CAD build for the part. Positions are in the model's coordinates, mm. A direction names the side the tool comes from. Coordinates: 2 decimals unless noted, no trailing zeros.
from build123d import *

# Parameters (mm, degrees)
SKIZZE2_W                            = 24
SKIZZE2_H                            = 26
SCHNITT_LINEAR_AUSTRAGEN1_DEPTH      = 62.5
KREISMUSTER1_COUNT                   = 8
SKIZZE3_R                            = 1.65
SCHNITT_LINEAR_AUSTRAGEN2_DEPTH      = 29.067398613
KREISMUSTER2_COUNT                   = 8
SKIZZE4_R                            = 1.25
SCHNITT_LINEAR_AUSTRAGEN3_DEPTH      = 6
SCHNITT_LINEAR_AUSTRAGEN3_DEPTH_BACK = 27.0000001
SCHNITT_LINEAR_AUSTRAGEN4_REACH      = 42
SKIZZE5_W                            = 3
SKIZZE5_H                            = 36.82390528
SKIZZE6_W                            = 7.166939891
SKIZZE6_H                            = 30
SCHNITT_LINEAR_AUSTRAGEN5_DEPTH      = 2.0000001
SCHNITT_LINEAR_AUSTRAGEN5_DEPTH_BACK = 2.5
SKIZZE12_R                           = 1.25
SCHNITT_LINEAR_AUSTRAGEN6_DEPTH      = 10
SCHNITT_LINEAR_AUSTRAGEN7_REACH      = 39.5


with BuildPart() as part:
    # Skizze1 → Rotation1 (revolve)
    with BuildSketch(Plane.XY):
        Polygon((-53, -1), (-53, 40), (-60, 40), (-60, 11), (-61.5, 11), (-61.5, 8), (-55, 8), (-55, 3.600622615), (-58, 1.5), (-58, 0), (-54, 0), (-54, -1), align=None)
    revolve(axis=Axis((0, 0, 0), (0, 1, 0)))

    # Skizze2 → Schnitt-Linear austragen1 (cut, through all)
    with BuildSketch(Plane(origin=(0, 0, 0), x_dir=(0, 0, -1), z_dir=(1, 0, 0))):
        with Locations((0, 27)):
            Rectangle(SKIZZE2_W, SKIZZE2_H)
    schnitt_linear_austragen1 = extrude(amount=-SCHNITT_LINEAR_AUSTRAGEN1_DEPTH, mode=Mode.SUBTRACT)

    # Kreismuster1: Schnitt-Linear austragen1 ×8 about axis
    kreismuster1_axis = Axis((0, 0, 0), (0, 1, 0))
    for i in range(1, KREISMUSTER1_COUNT):
        add(schnitt_linear_austragen1.rotate(kreismuster1_axis, i * 360 / KREISMUSTER1_COUNT), mode=Mode.SUBTRACT)

    # Skizze3 → Schnitt-Linear austragen2 (cut, through all)
    with BuildSketch(Plane(origin=(20.009071561, 0, 48.306171934), x_dir=(-0.923879533, 0, 0.382683432), z_dir=(-0.382683432, 0, -0.923879533))):
        with Locations((0, 25)):
            Circle(SKIZZE3_R)
    schnitt_linear_austragen2 = extrude(amount=-SCHNITT_LINEAR_AUSTRAGEN2_DEPTH, mode=Mode.SUBTRACT)

    # Kreismuster2: Schnitt-Linear austragen2 ×8 about axis
    kreismuster2_axis = Axis((0, 0, 0), (0, -1, 0))
    for i in range(1, KREISMUSTER2_COUNT):
        add(schnitt_linear_austragen2.rotate(kreismuster2_axis, i * 360 / KREISMUSTER2_COUNT), mode=Mode.SUBTRACT)

    # Skizze4 → Schnitt-Linear austragen3 (cut, two sides)
    with BuildSketch(Plane(origin=(0, 14, 0), x_dir=(-1, 0, 0), z_dir=(0, -1, 0))) as schnitt_linear_austragen3_sk:
        with Locations((0, 57)):
            Circle(SKIZZE4_R)
        with Locations((40.305086528, 40.305086528)):
            Circle(SKIZZE4_R)
        with Locations((57, 0)):
            Circle(SKIZZE4_R)
        with Locations((40.305086528, -40.305086528)):
            Circle(SKIZZE4_R)
        with Locations((0, -57)):
            Circle(SKIZZE4_R)
        with Locations((-40.305086528, -40.305086528)):
            Circle(SKIZZE4_R)
        with Locations((-57, 0)):
            Circle(SKIZZE4_R)
        with Locations((-40.305086528, 40.305086528)):
            Circle(SKIZZE4_R)
    extrude(amount=SCHNITT_LINEAR_AUSTRAGEN3_DEPTH, mode=Mode.SUBTRACT)
    extrude(schnitt_linear_austragen3_sk.sketch, amount=-SCHNITT_LINEAR_AUSTRAGEN3_DEPTH_BACK, mode=Mode.SUBTRACT)

    # Skizze5 → Schnitt-Linear austragen4 (cut, up to next)
    with BuildSketch(Plane.XZ, mode=Mode.PRIVATE) as schnitt_linear_austragen4_sk1:
        with Locations((56.5, 0)):
            Rectangle(SKIZZE5_W, SKIZZE5_H)
    schnitt_linear_austragen4_tool1 = extrude(schnitt_linear_austragen4_sk1.sketch, amount=-SCHNITT_LINEAR_AUSTRAGEN4_REACH, mode=Mode.PRIVATE) & part.part
    add(schnitt_linear_austragen4_tool1.solids().sort_by_distance((56.5, 0, 0))[0], mode=Mode.SUBTRACT)

    # Skizze6 → Schnitt-Linear austragen5 (cut, two sides)
    with BuildSketch(Plane.XZ) as schnitt_linear_austragen5_sk:
        with Locations((-54.416530055, 0)):
            Rectangle(SKIZZE6_W, SKIZZE6_H)
    extrude(amount=SCHNITT_LINEAR_AUSTRAGEN5_DEPTH, mode=Mode.SUBTRACT)
    extrude(schnitt_linear_austragen5_sk.sketch, amount=-SCHNITT_LINEAR_AUSTRAGEN5_DEPTH_BACK, mode=Mode.SUBTRACT)

    # Skizze12 → Schnitt-Linear austragen6 (cut)
    with BuildSketch(Plane(origin=(0, 40, 0), x_dir=(1, 0, 0), z_dir=(0, 1, 0))):
        with Locations((-51.737253821, -21.430272212)):
            Circle(SKIZZE12_R)
        with Locations((-51.737253821, 21.430272212)):
            Circle(SKIZZE12_R)
        with Locations((-21.430272212, 51.737253821)):
            Circle(SKIZZE12_R)
        with Locations((21.430272212, 51.737253821)):
            Circle(SKIZZE12_R)
        with Locations((51.737253821, 21.430272212)):
            Circle(SKIZZE12_R)
        with Locations((51.737253821, -21.430272212)):
            Circle(SKIZZE12_R)
        with Locations((21.430272212, -51.737253821)):
            Circle(SKIZZE12_R)
        with Locations((-21.430272212, -51.737253821)):
            Circle(SKIZZE12_R)
    extrude(amount=-SCHNITT_LINEAR_AUSTRAGEN6_DEPTH, mode=Mode.SUBTRACT)

    # Skizze13 → Schnitt-Linear austragen7 (cut, up to next)
    with BuildSketch(Plane.XZ.offset(-2.5), mode=Mode.PRIVATE) as schnitt_linear_austragen7_sk1:
        with BuildLine():
            Line((-53.5, -5), (-53.5, 5))
            ThreePointArc((-53.5, 5), (-49.5, 9), (-45.5, 5))
            Line((-45.5, 5), (-45.5, -5))
            ThreePointArc((-45.5, -5), (-49.5, -9), (-53.5, -5))
        make_face()
    schnitt_linear_austragen7_tool1 = extrude(schnitt_linear_austragen7_sk1.sketch, amount=-SCHNITT_LINEAR_AUSTRAGEN7_REACH, mode=Mode.PRIVATE) & part.part
    add(schnitt_linear_austragen7_tool1.solids().sort_by_distance((-49.5, 2.5, 0))[0], mode=Mode.SUBTRACT)


solid = part.part
1) Drill centre lines: probe 1 along Z at (x, y) = (20.5, 34); probe 2 along Y at (x, z) = (-40.5, 34.5); probe 3 along Y at (x, z) = (-1.5, -54.5). Where is each one in solid material? Low to high.
2) Pin check, flat tips, straight feed: P1, Ø2, axis at y = 24, z = 47.5, coming from the +X side; P2, Ø12, axis at y = 21, z = 12.5, coming from the -X side; P3, Ø3, axis at x = 22, y = 5.5, coming from the -Z side. Stop position of each tip, or through.
3) Which spindle directions (+Z, -Z, +X, -X, +Y, -Y) get a long thin tool onto all of the face, cutting with end or side? Do faces 1 (the flat face through (-12, 27, -55)), 2 (the flat face through (-54, 2.5, 0)), 3 (the flat face through (55, 1, 0)), 4 (the flat face through (-50, 0, -21)). Say none if no direction does.
4) Two-plate mould, pull along Z, no slides. Class faces 5 (the cylindrical face through (-28.38, 9.48, -54.56)), 6 (the flat face through (20, 40, -52)), 7 (the flat face through (-55, 14, 0)): released by +Z, released by -Z, zero draft, split by the parting line, or undercut.
5) Slice it at A-A (y = 21.5). Give the number of separate pieces and of enclosed holes in the cut face, plus the area to 3 significant figures.
Worked out:
1. probe 1: z = -56.39 to -52.57, -50.9 to -48.87, 48.87 to 50.9, 52.57 to 56.39
1. probe 2: y = -1 to 14
1. probe 3: y = 0 to 14
2. P1: stops at x = 31.53
2. P2: stops at x = -58.79
2. P3: stops at z = -51.04
3. face 1: +Z, -Z, +Y
3. face 2: -X, -Y
3. face 3: +Z, -Z, +X, -Y
3. face 4: -Y
4. face 5: split by the parting line
4. face 6: zero draft
4. face 7: undercut
5. separate pieces: 8
5. enclosed holes: 0
5. area: 1,130 mm2
